The model under review builds one solid part; all positions refer to its coordinate system, in mm. Face numbers are marked on the shaded views. A direction names the side the tool comes from. Coordinates: 2 decimals unless noted, no trailing zeros. Order: outer loops, then holes, each group sorted by start corner. A loop starts at its lowest first (then second) coordinate and runs counter-clockwise, first axis right, second up. Notation, with made-up numbers: (36.5, 76.5) - (89.5, 76.5) arc R12 cw to (89.5, 98.5) - close; hole circle Ø7 at (-15, -26.5). An arc over 180 degrees is marked (long way). Answer in a Markdown table with one row per item.
```python
from build123d import *

# Parameters (mm, degrees)
SKETCH1_W           = 15.5
SKETCH1_H           = 11
BOSS_EXTRUDE1_DEPTH = 1.6
BOSS_EXTRUDE2_DEPTH = 1.6
SKETCH3_W           = 15.5
SKETCH3_H           = 2.7
BOSS_EXTRUDE3_DEPTH = 2.7
SKETCH4_W           = 40.2
SKETCH4_H           = 1.6
BOSS_EXTRUDE4_DEPTH = 60.3
SKETCH5_W           = 30.1
SKETCH5_H           = 9.2
BOSS_EXTRUDE5_DEPTH = 12.1
SKETCH6_R           = 2
CUT_EXTRUDE1_DEPTH  = 2
LPATTERN1_COUNT     = 6
LPATTERN1_PITCH     = 5


with BuildPart() as part:
    # Sketch1 → Boss-Extrude1 (new body)
    with BuildSketch(Plane(origin=(0, 0, 0), x_dir=(1, 0, 0), z_dir=(0, 1, 0))):
        with Locations((7.75, -5.5)):
            Rectangle(SKETCH1_W, SKETCH1_H)
    extrude(amount=BOSS_EXTRUDE1_DEPTH)

    # Sketch2 → Boss-Extrude2 (add, through all)
    with BuildSketch(Plane(origin=(0, 1.6, 0), x_dir=(1, 0, 0), z_dir=(0, 1, 0))):
        with BuildLine():
            Line((-1.75, -4), (-1.75, -2.6))
            ThreePointArc((-1.75, -2.6), (-4.65, -5.5), (-1.75, -8.4))
            Line((-1.75, -8.4), (-1.75, -7))
            ThreePointArc((-1.75, -7), (-3.25, -5.5), (-1.75, -4))
        make_face()
        with BuildLine():
            ThreePointArc((0, -3.187533784), (-0.827002716, -2.750804479), (-1.75, -2.6))
            Line((-1.75, -2.6), (-1.75, -4))
            ThreePointArc((-1.75, -4), (-0.689339828, -4.439339828), (-0.25, -5.5))
            ThreePointArc((-0.25, -5.5), (-0.689339828, -6.560660172), (-1.75, -7))
            Line((-1.75, -7), (-1.75, -8.4))
            ThreePointArc((-1.75, -8.4), (-0.827002716, -8.249195521), (0, -7.812466216))
            Line((0, -7.812466216), (0, -3.187533784))
        make_face()
        with BuildLine():
            Line((0, -2.6), (-1.75, -2.6))
            ThreePointArc((-1.75, -2.6), (-0.827002716, -2.750804479), (0, -3.187533784))
            Line((0, -3.187533784), (0, -2.6))
        make_face()
        with BuildLine():
            ThreePointArc((0, -7.812466216), (-0.827002716, -8.249195521), (-1.75, -8.4))
            Line((-1.75, -8.4), (0, -8.4))
            Line((0, -8.4), (0, -7.812466216))
        make_face()
        with BuildLine():
            ThreePointArc((20.15, -5.5), (19.300609665, -3.449390335), (17.25, -2.6))
            Line((17.25, -2.6), (17.25, -4))
            ThreePointArc((17.25, -4), (18.310660172, -4.439339828), (18.75, -5.5))
            ThreePointArc((18.75, -5.5), (18.310660172, -6.560660172), (17.25, -7))
            Line((17.25, -7), (17.25, -8.4))
            ThreePointArc((17.25, -8.4), (19.300609665, -7.550609665), (20.15, -5.5))
        make_face()
        with BuildLine():
            Line((17.25, -4), (17.25, -2.6))
            ThreePointArc((17.25, -2.6), (16.327002716, -2.750804479), (15.5, -3.187533784))
            Line((15.5, -3.187533784), (15.5, -7.812466216))
            ThreePointArc((15.5, -7.812466216), (16.327002716, -8.249195521), (17.25, -8.4))
            Line((17.25, -8.4), (17.25, -7))
            ThreePointArc((17.25, -7), (15.75, -5.5), (17.25, -4))
        make_face()
        with BuildLine():
            Line((17.25, -2.6), (15.5, -2.6))
            Line((15.5, -2.6), (15.5, -3.187533784))
            ThreePointArc((15.5, -3.187533784), (16.327002716, -2.750804479), (17.25, -2.6))
        make_face()
        with BuildLine():
            Line((15.5, -7.812466216), (15.5, -8.4))
            Line((15.5, -8.4), (17.25, -8.4))
            ThreePointArc((17.25, -8.4), (16.327002716, -8.249195521), (15.5, -7.812466216))
        make_face()
    extrude(amount=-BOSS_EXTRUDE2_DEPTH)

    # Sketch3 → Boss-Extrude3 (add)
    with BuildSketch(Plane(origin=(0, 1.6, 0), x_dir=(1, 0, 0), z_dir=(0, 1, 0))):
        with Locations((7.75, -9.15)):
            Rectangle(SKETCH3_W, SKETCH3_H)
    extrude(amount=BOSS_EXTRUDE3_DEPTH)

    # Sketch4 → Boss-Extrude4 (add)
    with BuildSketch(Plane(origin=(0, 4.3, 0), x_dir=(1, 0, 0), z_dir=(0, 1, 0))):
        with Locations((7.75, -10.112281479)):
            Rectangle(SKETCH4_W, SKETCH4_H)
    extrude(amount=BOSS_EXTRUDE4_DEPTH)

    # Sketch5 → Boss-Extrude5 (add)
    with BuildSketch(Plane(origin=(0, 0, 9.312281479), x_dir=(-1, 0, 0), z_dir=(0, 0, -1))):
        with Locations((-6.7, 45.3)):
            Rectangle(SKETCH5_W, SKETCH5_H)
    extrude(amount=BOSS_EXTRUDE5_DEPTH)

    # Sketch6 → Cut-Extrude1 (cut)
    with BuildSketch(Plane(origin=(0, 0, -2.787718521), x_dir=(-1, 0, 0), z_dir=(0, 0, -1))):
        with Locations((-19.35, 45.7)):
            Circle(SKETCH6_R)
    cut_extrude1 = extrude(amount=-CUT_EXTRUDE1_DEPTH, mode=Mode.SUBTRACT)

    # LPattern1: Cut-Extrude1 ×6
    with Locations(*[(-i * LPATTERN1_PITCH, 0, 0) for i in range(1, LPATTERN1_COUNT)]):
        add(cut_extrude1, mode=Mode.SUBTRACT)


solid = part.part
```
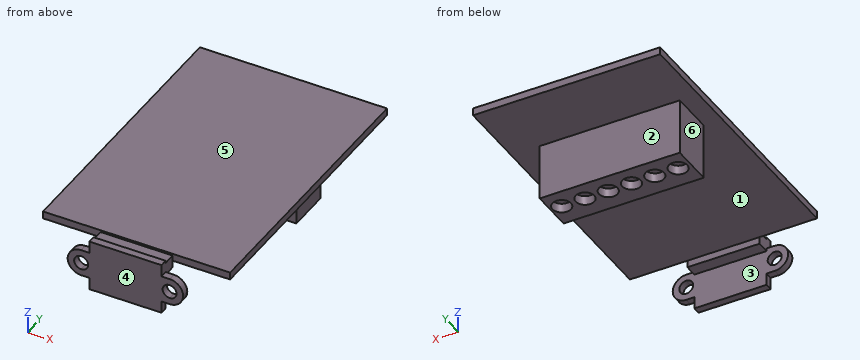
Item 1: Tool access review of the marked faces 5 and 6: name each direction out of +Z, -Z, +X, -X, +Y, -Y from which nothing blocks a thin tool from reaching the whole face with its end or side.
Check values:
| item | result |
|---|---|
| face 5 | +Z, +X, -X, +Y |
| face 6 | -Z, -X, +Y, -Y |
Item 2: We need section D-D, the plane x = -5.65. Write out the cut boundary in (y, z).
Check values:
| item | result |
|---|---|
| outline | (4.3, 9.31) - (40.7, 9.31) - (40.7, -2.79) - (43.7, -2.79) - (43.7, -0.79) - (47.7, -0.79) - (47.7, -2.79) - (49.9, -2.79) - (49.9, 9.31) - (64.6, 9.31) - (64.6, 10.91) - (4.3, 10.91) - close |
Item 3: Mouldability with a two-part tool opening along Y and no side actions: class the marked faces 1, 2, 3 and 4 as +Y half, -Y half, draft (parallel to the pull), parting line (faces both ways), or undercut.
Check values:
| item | result |
|---|---|
| face 1 | undercut |
| face 2 | +Y half |
| face 3 | undercut |
| face 4 | -Y half |
Item 4: We need section B-B, the plane y = 49. Write out the cut boundary in (x, z).
Check values:
| item | result |
|---|---|
| outline | (-12.35, 9.31) - (-8.35, 9.31) - (-8.35, -2.79) - (21.75, -2.79) - (21.75, 9.31) - (27.85, 9.31) - (27.85, 10.91) - (-12.35, 10.91) - close |
Item 5: We need section A-A, the plane z = 1.25. Write out the cut boundary in (x, y).
Check values:
| item | result |
|---|---|
| outline | (-8.35, 40.7) - (21.75, 40.7) - (21.75, 49.9) - (-8.35, 49.9) - close; (0, 0) - (15.5, 0) - (15.5, 1.6) - (0, 1.6) - close |
Item 6: To check wall thickness, follow line 1 (Y direction, x = 9.35, z = -2.4); line 2 (Y direction, x = 2, z = 4.5); line 3 (Y direction, x = -6.5, z = 2.75). State the ranges of each line that lie inside material, in increasing order. Write a range as from..to.
Check values:
| item | result |
|---|---|
| line 1 | 40.7..43.7, 47.7..49.9 |
| line 2 | 0..1.6, 40.7..49.9 |
| line 3 | 40.7..49.9 |
Item 7: Clearance check with flat-ended pins moving along their axes: pin 1 Ø8 at (x, y) = (6, 48) entering from +Z; pin 2 Ø4 at (x, z) = (11.5, 9.5) entering from -Y; pin 3 Ø0.8 at (y, z) = (1, 1.5) entering from -X; pin 4 Ø5 at (x, y) = (20.5, 26) entering from -Z. State where each tip first meets the part, or that it passes through.
Check values:
| item | result |
|---|---|
| pin 1 | z = 10.91 |
| pin 2 | y = 0 |
| pin 3 | x = 0 |
| pin 4 | z = 9.31 |
Item 8: We need section C-C, the plane x = 14.35. Write out the cut boundary in (y, z).
Check values:
| item | result |
|---|---|
| outline | (0, 0) - (1.6, 0) - (1.6, 7.8) - (4.3, 7.8) - (4.3, 9.31) - (40.7, 9.31) - (40.7, -2.79) - (43.7, -2.79) - (43.7, -0.79) - (47.7, -0.79) - (47.7, -2.79) - (49.9, -2.79) - (49.9, 9.31) - (64.6, 9.31) - (64.6, 10.91) - (4.3, 10.91) - (4.3, 10.5) - (1.6, 10.5) - (1.6, 11) - (0, 11) - close |
